```python
from build123d import *

# Parameters (mm, degrees)
F0_W     = 70
F0_H     = 50
F1_DEPTH = 10
F2_SIZE2 = 6.9282032303
F2_SIZE  = 12
F3_R     = 16
F4_DEPTH = 2.5
F5_W     = 69
F5_H     = 12.8564064606
F6_DEPTH = 2


with BuildPart() as f1:
    # F0 (on Top) → F1 (new body)
    with BuildSketch(Plane.XY):
        with Locations((5.1442100421, 5.2647431195)):
            Rectangle(F0_W, F0_H)
    extrude(amount=F1_DEPTH)

    # F2
    f2_edges = [f1.edges().sort_by_distance(p)[0] for p in [
        (5.14421, -19.735257, 10),
    ]]
    f2_side = f1.faces().sort_by_distance((5.14421, 5.264743, 10))[0]
    chamfer(f2_edges, length=F2_SIZE, length2=F2_SIZE2, reference=f2_side)

    # F3 (on face) → F4 (cut)
    with BuildSketch(Plane.XY.offset(10)):
        with Locations((5.1442100421, 11.2647431195)):
            Circle(F3_R)
    extrude(amount=-F4_DEPTH, mode=Mode.SUBTRACT)

    # F5 (on face) → F6 (cut)
    with BuildSketch(Plane(origin=(0, -6.2639412391, 10.8494644817), x_dir=(1, 0, 0), z_dir=(0, -0.5, 0.8660254038))):
        with Locations((5.1442100421, -8.6271321936)):
            Rectangle(F5_W, F5_H)
    extrude(amount=-F6_DEPTH, mode=Mode.SUBTRACT)


solid = f1.part
```
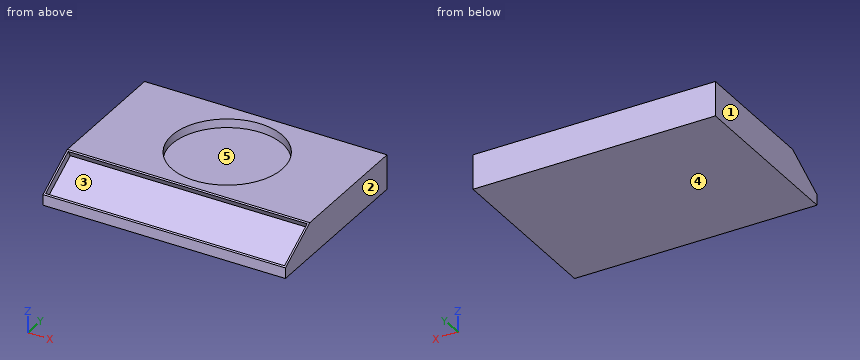
For this review, take the finished solid that the model builds, in its own axes (mm). Face numbers are marked on the shaded views. A direction names the side the tool comes from. Coordinates: 2 decimals unless noted, no trailing zeros. Order: outer loops, then holes, each group sorted by start corner. A loop starts at its lowest first (then second) coordinate and runs counter-clockwise, first axis right, second up. Notation, with made-up numbers: (1.5, -23.75) - (50.5, -23.75) arc R14 cw to (50.5, -18.75) - close; hole circle Ø10 at (77.25, 20.25). An arc over 180 degrees is marked (long way). Answer as a JSON object with one key per item and string values. Group by question number.
1. We need section A-A on x = -17.5. State the section outline as (y, z) points.
2. For probe 1 along Y at (x, z) = (-8, 2.75); probe 2 along X at (y, z) = (-15, 5); probe 3 along Y at (x, z) = (14, 8.5), list the stretches that pass through material, from the lowest coordinate up.
3. We need section C-C on z = 8.75. State the section outline as (x, y) points.
4. We need section B-B on y = -13. State the section outline as (x, z) points, then the cut area to 3 significant figures.
5. The part is to be moulded in two halves that separate along X. For the marked faces 1, 2 and 3, say which applies: pulls with the +X half, pulls with the -X half, needs draft (parallel to the pull), parting line crosses it, or undercut.
6. For the marked faces 4 and 5, list the 3-axis set-ups (+Z, -Z, +X, -X, +Y, -Y) from which the entire face can be reached by the end or side of a thin tool; tool diameter is ignored.
7. Clearance check with a flat-ended pin moving along its axis: P1, Ø1.5, axis at x = 1, z = 7, coming from the -Y side. State where the tip first meets the part, or that it passes through.
8. We need section D-D on z = 5.25. State the section outline as (x, y) points, then the cut area to 3 significant figures.
Final values:
{
 "1": {"outline": "(-19.74, 0) - (30.26, 0) - (30.26, 10) - (-7.74, 10) - (-8.17, 9.75) - (-7.17, 8.02) - (-18.3, 1.59) - (-19.3, 3.32) - (-19.74, 3.07) - close"},
 "2": {"probe 1": "-19.74 to -18.97, -16.29 to 30.26", "probe 2": "-29.86 to -29.36, 39.64 to 40.14", "probe 3": "-7.45 to -2.06, 24.59 to 30.26"},
 "3": {"outline": "(-29.86, -9.9) - (-29.36, -9.9) - (-29.36, -7.59) - (39.64, -7.59) - (39.64, -9.9) - (40.14, -9.9) - (40.14, 30.26) - (-29.86, 30.26) - close; hole circle Ø32 at (5.14, 11.26)"},
 "4": {"outline": "(-29.86, 0) - (40.14, 0) - (40.14, 6.96) - (39.64, 6.96) - (39.64, 4.65) - (-29.36, 4.65) - (-29.36, 6.96) - (-29.86, 6.96) - close", "area": "328 mm²"},
 "5": {"face 1": "pulls with the -X half", "face 2": "pulls with the +X half", "face 3": "undercut"},
 "6": {"face 4": "-Z, +X, -X, +Y, -Y", "face 5": "+Z"},
 "7": {"P1": "y = -10.23"},
 "8": {"outline": "(-29.86, -15.96) - (-29.36, -15.96) - (-29.36, -11.96) - (39.64, -11.96) - (39.64, -15.96) - (40.14, -15.96) - (40.14, 30.26) - (-29.86, 30.26) - close", "area": "2,960 mm²"}
}
